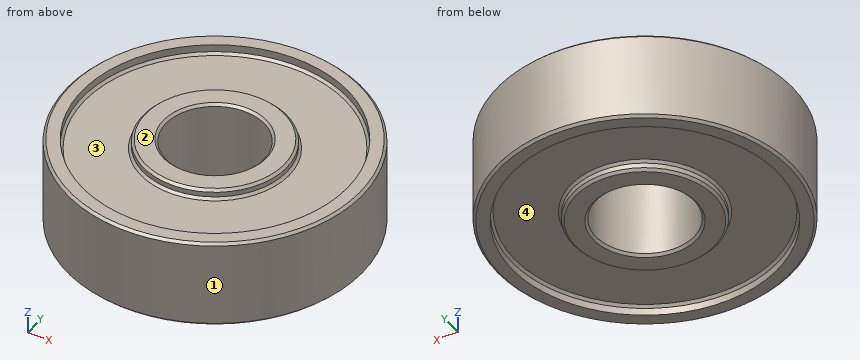
from build123d import *

# Parameters (mm, degrees)
SKETCH_1_R          = 15
EXTRUDE_1_DEPTH     = 9
SKETCH_2_R          = 5
CUT_EXTRUDE_1_DEPTH = 10
SKETCH_3_W          = 6.2
SKETCH_3_H          = 1
CHAMFER_1_SIZE      = 0.25


with BuildPart() as part:
    # Эскиз1 → Бобышка-Вытянуть1 (new body)
    with BuildSketch(Plane.XY):
        Circle(SKETCH_1_R)
    extrude(amount=EXTRUDE_1_DEPTH)

    # Эскиз2 → Вырез-Вытянуть1 (cut, through all)
    with BuildSketch(Plane(origin=(0, 0, 0), x_dir=(-1, 0, 0), z_dir=(0, 0, -1))):
        Circle(SKETCH_2_R)
    extrude(amount=-CUT_EXTRUDE_1_DEPTH, mode=Mode.SUBTRACT)

    # Эскиз3 → Вырез-Повернуть1 (revolve, cut)
    with BuildSketch(Plane(origin=(0, 0, 0), x_dir=(1, 0, 0), z_dir=(0, 1, 0))):
        with Locations((10.4, -8.5)):
            Rectangle(SKETCH_3_W, SKETCH_3_H)
        with Locations((10.4, -0.5)):
            Rectangle(SKETCH_3_W, SKETCH_3_H)
    revolve(axis=Axis((0, 0, 9), (0, 0, -1)), mode=Mode.SUBTRACT)

    # Фаска1
    chamfer_1_edges = [part.edges().sort_by_distance(p)[0] for p in [
        (-7.3, 0, 9),
        (-7.3, 0, 8),
        (-13.5, 0, 8),
        (-7.3, 0, 1),
        (-13.5, 0, 1),
        (-7.3, 0, 0),
        (-15, 0, 0),
        (-15, 0, 9),
        (5, 0, 9),
        (5, 0, 0),
    ]]
    chamfer(chamfer_1_edges, length=CHAMFER_1_SIZE)


solid = part.part
The listing builds one solid part. Answer for the finished solid, in the listing's coordinates (mm). Face numbers are marked on the shaded views. Round coordinates to 2 decimals unless told otherwise and drop trailing zeros. Loops run counter-clockwise (first coordinate to the right, second up) from the corner with the lowest first, then second, coordinate; pieces in that order, holes last. Notation, with made-up numbers: M 67.25,80 L 115.25,80 A23 cw 115.25,113 Z; hole C 10,21.5 d1. An arc over 180 degrees is marked long. Return JSON: item names as keys, results as strings.
Q1. Each of these flat-tipped pins is pushed along its axis until it touches: pin 1 Ø1 at (y, z) = (5, 6) entering from +X; pin 2 Ø2 at (x, y) = (1.5, -6) entering from -Z; pin 3 Ø5 at (y, z) = (3, 1.5) entering from -X; pin 4 Ø3 at (x, y) = (8.5, 2.5) entering from +Z. Where does it stop, or does it pass through?
Results list:
{"pin 1": "stops at x = 14.31", "pin 2": "stops at z = 0", "pin 3": "stops at x = -14.99", "pin 4": "stops at z = 8.19"}
Q2. Find the intervals of material crossed by line 1 along Y through (x, z) = (0, 8.65); line 2 along Y through (x, z) = (0, 4); line 3 along Y through (x, z) = (0, 8.8), in increasing order. Write a range as from..to.
Results list:
{"line 1": "y = -15..-13.5, -7.3..-5, 5..7.3, 13.5..15", "line 2": "y = -15..-5, 5..15", "line 3": "y = -14.95..-13.5, -7.25..-5.05, 5.05..7.25, 13.5..14.95"}
Q3. Find section A-A, the plane z = 6.25. Determine the outline of the cut face in (x, y).
Results list:
{"outline": "C 0,0 d30; hole C 0,0 d10"}
Q4. The mould has two halves that part along Y. Classify the marked faces 1, 2, 3 and 4: released by +Y, released by -Y, zero draft, split by the parting line, or undercut.
Results list:
{"face 1": "split by the parting line", "face 2": "zero draft", "face 3": "undercut", "face 4": "undercut"}
